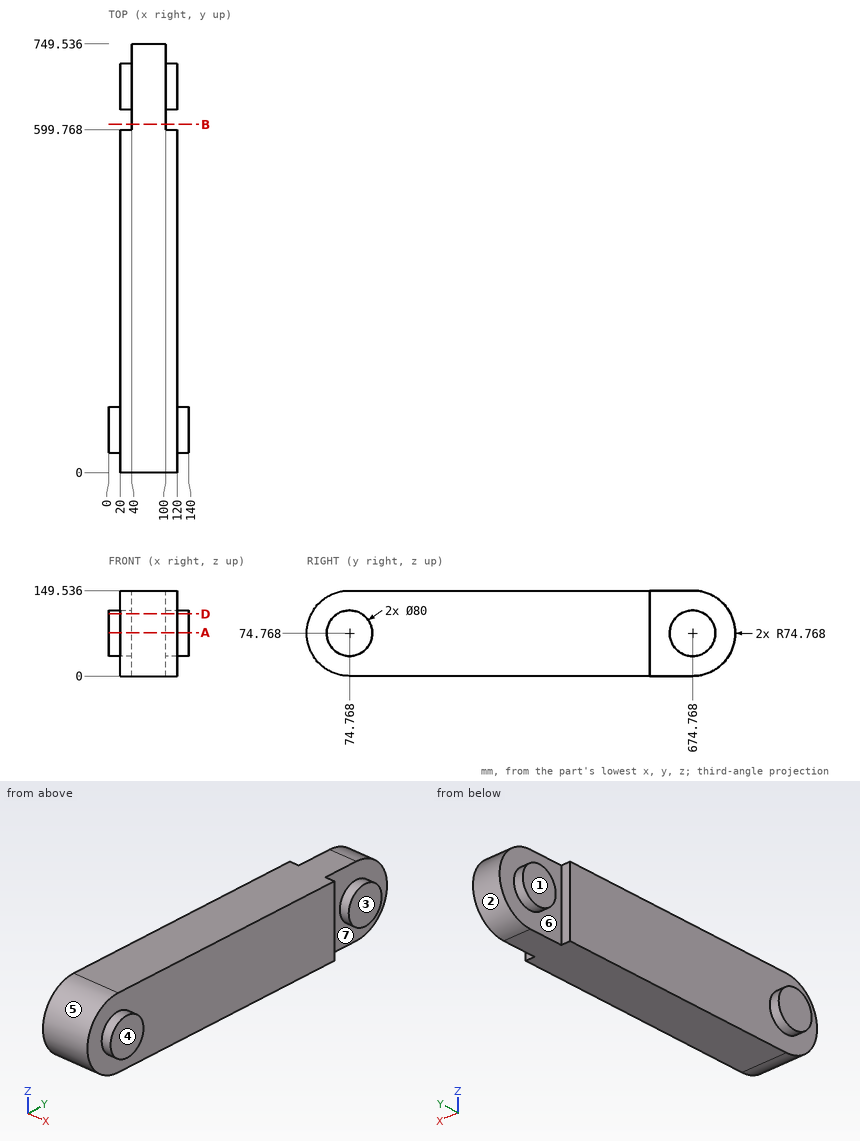
Answer from the drawing. Dimensions are ordinates in mm from the lowest x, y and z of the part. A direction names the side the tool comes from. Round coordinates to 2 decimals unless told otherwise and drop trailing zeros. Order: outer loops, then holes, each group sorted by start corner. A loop starts at its lowest first (then second) coordinate and runs counter-clockwise, first axis right, second up. Notation, with made-up numbers: (-14.75, 61) - (34.25, 61) arc R5 cw to (34.25, 65) - close; hole circle Ø2 at (58, -11.5). An arc over 180 degrees is marked (long way). Put each result on its own line as item: value. Start each with the question number.
(1) Find section D-D (z = 108.5). Give the vertices of the cut face in (x, y) (1 decimal), plus the area to 3 significant figures.
(2) Given P1, Ø6, axis at y = 137, z = 108, coming from the +X side; P2, Ø10, axis at x = 29, z = 57.5, coming from the +Y side; P3, Ø1, axis at x = 61, z = 32, coming from the -Y side (1 decimal), each flat-ended and moving along its own axis, determine where each tip first touches the part or whether it passes through.
(3) Find section A-A (z = 76). Give the vertices of the cut face in (x, y) (1 decimal).
(4) For the marked faces 1, 2 and 3, determine the directions among +Z, -Z, +X, -X, +Y, -Y from which every point of the face is accessible in a straight line to the end or side of a thin tool.
(5) Find section B-B (y = 609). Give the vertices of the cut face in (x, z) (1 decimal), plus the area to 3 significant figures.
(6) Straight lines are drawn through the part: probe 1 along Y at (x, z) = (108, 74) (1 decimal); probe 2 along X at (y, z) = (154, 58.5); probe 3 along Y at (x, z) = (31, 59.5) (1 decimal). For each, find the intervals that lie inside material, in ascending order. Write a range as from..to.
(7) Determine the mould class of the marked faces 4, 5, 6 and 7 for opening direction Y: released by +Y, released by -Y, zero draft, split by the parting line, or undercut.
Reply:
1. outline: (0, 53.3) - (20, 53.3) - (20, 8) - (120, 8) - (120, 53.3) - (140, 53.3) - (140, 96.3) - (120, 96.3) - (120, 599.8) - (100, 599.8) - (100, 653.3) - (120, 653.3) - (120, 696.3) - (100, 696.3) - (100, 741.5) - (40, 741.5) - (40, 696.3) - (20, 696.3) - (20, 653.3) - (40, 653.3) - (40, 599.8) - (20, 599.8) - (20, 96.3) - (0, 96.3) - close
1. area: 71,100 mm^2
2. P1: x = 120
2. P2: y = 712.84
2. P3: y = 13.1
3. outline: (0, 34.8) - (20, 34.8) - (20, 0) - (120, 0) - (120, 34.8) - (140, 34.8) - (140, 114.7) - (120, 114.7) - (120, 599.8) - (100, 599.8) - (100, 634.8) - (120, 634.8) - (120, 714.7) - (100, 714.7) - (100, 749.5) - (40, 749.5) - (40, 714.7) - (20, 714.7) - (20, 634.8) - (40, 634.8) - (40, 599.8) - (20, 599.8) - (20, 114.7) - (0, 114.7) - close
4. face 1: +Z, -Z, -X, +Y
4. face 2: +X, -X, +Y
4. face 3: +Z, -Z, +X, +Y
5. outline: (40, 0) - (100, 0) - (100, 149.5) - (40, 149.5) - close
5. area: 8,970 mm^2
6. probe 1: 0..599.8, 634.8..714.8
6. probe 2: 20..120
6. probe 3: 1.6..599.8, 637.8..711.7
7. face 4: zero draft
7. face 5: released by -Y
7. face 6: undercut
7. face 7: undercut
